Geometry: final body of the model. Coordinates: model frame, mm. Face numbers are marked on the shaded views. A direction names the side the tool comes from. Round coordinates to 2 decimals unless told otherwise and drop trailing zeros. Answer in a Markdown table with one row per item.
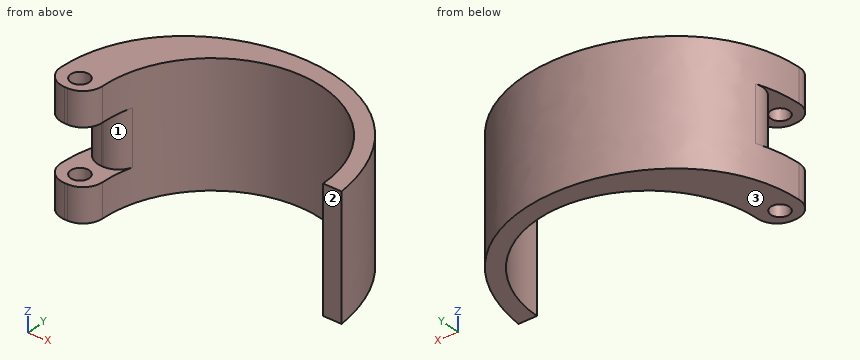
```python
from build123d import *

# Parameters (mm, degrees)
PAD_DEPTH       = 20
SKETCH005_R     = 1.5
POCKET_DEPTH    = 20.001
SKETCH008_W     = 19.422657
SKETCH008_H     = 9
POCKET002_DEPTH = 6
FILLET002_R     = 3.2


with BuildPart() as part:
    # Sketch → Pad (new body)
    with BuildSketch(Plane.XY):
        with BuildLine():
            Line((18, 0), (21, 0))
            add(Edge.make_bspline(
                [(21, 0), (18.005676, 31.142447), (-27.438789, 25.917835), (-24.780889, -2.8)],
                knots=[0, 0, 0, 0, 1, 1, 1, 1], degree=3))
            Line((-24.780889, -2.8), (-17.780889, -2.8))
            ThreePointArc((-17.780889, -2.8), (-1.40428, 17.945139), (18, 0))
        make_face()
    extrude(amount=PAD_DEPTH)

    # Sketch005 (on Face6 of Pad) → Pocket (cut, through all)
    with BuildSketch(Plane.XY.offset(20)):
        with Locations((-21.380889, 0)):
            Circle(SKETCH005_R)
    extrude(amount=-POCKET_DEPTH, mode=Mode.SUBTRACT)

    # Sketch008 (on Face6 of Pocket) → Pocket002 (cut)
    with BuildSketch(Plane.XZ.offset(2.8)):
        with Locations((-21.679914, 10)):
            Rectangle(SKETCH008_W, SKETCH008_H)
    extrude(amount=-POCKET002_DEPTH, mode=Mode.SUBTRACT)

    # Fillet002
    fillet002_edges = [part.edges().sort_by_distance(p)[0] for p in [
        (-17.713272, 3.2, 10),
        (-24.614915, 3.2, 10),
        (-24.780889, -2.8, 2.75),
        (-17.780889, -2.8, 2.75),
        (-17.780889, -2.8, 17.25),
        (-24.780889, -2.8, 17.25),
    ]]
    fillet(fillet002_edges, radius=FILLET002_R)


solid = part.part
```
Item 1: Set-up query: the marked faces 1, 2 and 3. Return all of +Z, -Z, +X, -X, +Y, -Y with unobstructed straight access to the full face (end or side cutting, diameter ignored); none if empty.
Ans:
| item | result |
|---|---|
| face 1 | -Y |
| face 2 | +Z, -Z, +X, -Y |
| face 3 | -Z, +X, -X, +Y, -Y |
Item 2: Ray query, L1, parallel to X at y = 6.5, z = 13; L2, parallel to Y at x = 8, z = 2.5; L3, parallel to X at y = 11, z = 9.25. Return the intervals inside material, ascending.
Ans:
| item | result |
|---|---|
| L1 | -23.65 to -16.79, 16.79 to 19.61 |
| L2 | 16.12 to 19.17 |
| L3 | -21.67 to -14.25, 14.25 to 17.48 |
Item 3: First-contact query: P1, Ø12, axis at y = 17.5, z = 5, coming from the +X side; P2, Ø3.5, axis at x = 19.5, z = 11, coming from the -Y side; P3, Ø10, axis at x = -11, z = 3, coming from the -Y side; P4, Ø2.5, axis at x = -21.38, y = 0, coming from the -Z side. Flat tips, straight axial feed; report the tip coordinate or a pass-through.
Ans:
| item | result |
|---|---|
| P1 | x = 17.16 |
| P2 | y = 0 |
| P3 | y = 8.25 |
| P4 | through |
